Autodesk Inventor part; units mm, degrees
ref_plane "YZ Plane" through (0, 0, 0) normal (1, 0, 0) x (0, 1, 0)
ref_plane "XZ Plane" through (0, 0, 0) normal (0, 1, 0) x (-1, 0, 0)
ref_plane "XY Plane" through (0, 0, 0) normal (0, 0, 1) x (1, 0, 0)
sketch "Sketch1" plane through (0, 0, 0) normal (0, 1, 0) x (-1, 0, 0)
  line L0 (-78, 78) -> (78, 78)
  line L1 (78, 78) -> (78, -78)
  line L2 (78, -78) -> (-78, -78)
  line L3 (-78, -78) -> (-78, 78)
  line L4 (-78, 78) -> (78, -78) construction
  line L5 (78, 78) -> (-78, -78) construction
  point P0 (0, 0)
  dimension "d0" = 156
  dimension "d1" = 156
extrude "Body" add sketch "Sketch1" along normal blind 156
sketch "Sketch2" plane through (78, 0, 78) normal (1, 0, 0) x (0, 0, -1)
  circle A0 centre (80, 80) radius 20
  point P0 (78, 0)
extrude "RotAxis" cut sketch "Sketch2" against normal through all
sketch "Sketch4" plane through (0, 156, 0) normal (0, 1, 0) x (1, 0, 0)
  circle A0 centre (0, 0) radius 20
extrude "CableHole" cut sketch "Sketch4" against normal through all
sketch "Sketch5" plane through (0, 0, 0) normal (0, -1, 0) x (1, 0, 0)
  point P0 (0, 0)
  point P1 (-58, 58)
  point P2 (-58, -58)
  point P3 (58, -58)
  point P4 (58, 58)
hole "BoltHoles" at (-58, 0, 58) at (-58, 0, -58) at (58, 0, -58) at (58, 0, 58) direction (0, 1, 0) diameter 6 depth 20 tip angle 118
properties part number "AxisConnector"
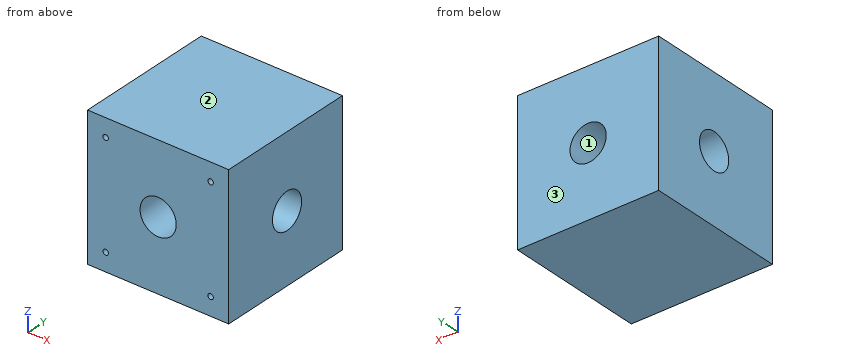
Verification items for the finished model (mm, model axes). Face numbers are marked on the shaded views. Coordinates: 2 decimals unless noted, no trailing zeros. Loops run counter-clockwise (first coordinate to the right, second up) from the corner with the lowest first, then second, coordinate; pieces in that order, holes last. Notation, with made-up numbers: (21.25, 29) -> (76.25, 29) arc R17 cw to (76.25, 49) -> close; hole circle Ø4 at (17.25, 27). An arc over 180 degrees is marked (long way). Put each result on its own line as item: value.
1. Gauge pin test, flat end, axial feed: P1, Ø3.5, axis at x = 58, z = 58, coming from the -Y side. Record the tip position at first contact, or that the pin passes through.
Result set:
P1: stops at y = 20.75
2. Section check A-A, the plane x = -34. Record the boundary of the cut face in (y, z).
Result set:
outline: (0, -78) -> (156, -78) -> (156, 78) -> (0, 78) -> close; hole circle Ø40 at (80, -2)
3. Thickness scan on line 1 (Z direction, x = -58, y = 4); line 2 (Y direction, x = 41, z = -2). Record the ranges inside material, lowest first.
Result set:
line 1: z = -78 to -61, -55 to 55, 61 to 78
line 2: y = 0 to 60, 100 to 156
4. Section check D-D, the plane x = 0. Record the boundary of the cut face in (y, z).
Result set:
outline: (0, -78) -> (156, -78) -> (156, -20) -> (88.72, -20) arc R20 cw to (71.28, -20) -> (0, -20) -> close; (0, 20) -> (156, 20) -> (156, 78) -> (0, 78) -> close
5. Section check B-B, the plane y = 67. Record the boundary of the cut face in (x, z), then the cut area to 3 significant figures.
Result set:
outline: (-78, -78) -> (78, -78) -> (78, -17.2) -> (10.21, -17.2) arc R20 cw to (-10.21, -17.2) -> (-78, -17.2) -> close; (-78, 13.2) -> (-15.03, 13.2) arc R20 cw to (15.03, 13.2) -> (78, 13.2) -> (78, 78) -> (-78, 78) -> close
area: 19,400 mm^2
6. Mould release check, pull along Z, two halves, no side actions. Record for the marked faces 1, 2 and 3: pulls with the +Z half, pulls with the -Z half, needs draft (parallel to the pull), parting line crosses it, or undercut.
Result set:
face 1: undercut
face 2: pulls with the +Z half
face 3: needs draft
7. Section check C-C, the plane z = 0. Record the boundary of the cut face in (x, y), then the cut area to 3 significant figures.
Result set:
outline: (-78, 0) -> (-20, 0) -> (-20, 60.1) -> (-78, 60.1) -> close; (-78, 99.9) -> (-20, 99.9) -> (-20, 156) -> (-78, 156) -> close; (20, 0) -> (78, 0) -> (78, 60.1) -> (20, 60.1) -> close; (20, 99.9) -> (78, 99.9) -> (78, 156) -> (20, 156) -> close
area: 13,500 mm^2
